from build123d import *

# Parameters (mm, degrees)
BASE_FLANGE1_DEPTH = 20
FILLET1_R          = 3
SKETCH2_R          = 1.5
CUT_EXTRUDE1_DEPTH = 3


# Sheet-metal steps are written as plain solids
with BuildPart() as part:
    # Sketch1 → Base-Flange1 (new body)
    with BuildSketch(Plane(origin=(0, 0, 0), x_dir=(0, 0, -1), z_dir=(1, 0, 0))):
        with BuildLine():
            Line((0, 0), (9.2634, 0))
            ThreePointArc((9.2634, 0), (9.784254855, 0.215745145), (10, 0.7366))
            Line((10, 0.7366), (10, 10))
            Line((10, 10), (13, 10))
            Line((13, 10), (13, 0.7366))
            ThreePointArc((13, 0.7366), (11.905575199, -1.905575199), (9.2634, -3))
            Line((9.2634, -3), (0, -3))
            Line((0, -3), (0, 0))
        make_face()
    extrude(amount=BASE_FLANGE1_DEPTH)

    # Fillet1
    fillet1_edges = [part.edges().sort_by_distance(p)[0] for p in [
        (20, -1.5, 0),
        (20, 10, -11.5),
        (0, -1.5, 0),
        (0, 10, -11.5),
    ]]
    fillet(fillet1_edges, radius=FILLET1_R)

    # Sketch2 → Cut-Extrude1 (cut)
    with BuildSketch(Plane(origin=(0, 0, -13), x_dir=(-1, 0, 0), z_dir=(0, 0, -1))):
        with Locations((-10, 2.5)):
            Circle(SKETCH2_R)
    extrude(amount=-CUT_EXTRUDE1_DEPTH, mode=Mode.SUBTRACT)


solid = part.part
Part model, mm, in its own coordinate system. A direction names the side the tool comes from. Coordinates: 2 decimals unless noted, no trailing zeros. Write each loop counter-clockwise with the first axis right and the second up, starting at its lowest first coordinate (ties: lowest second). Pieces come first, ordered by that corner, then holes. Notation, with made-up numbers: (-26, -30) - (4, -30) arc R18 ccw to (4, -26) - close; hole circle Ø9 at (-10, 2). An arc over 180 degrees is marked (long way). Put each result on its own line as item: value.
1. Band-saw the part on B-B (y = 2.5). Write the cut outline in (x, z), then the cut area to 3 significant figures.
Final values:
outline: (0, -13) - (8.5, -13) - (8.5, -10) - (0, -10) - close; (11.5, -13) - (20, -13) - (20, -10) - (11.5, -10) - close
area: 51.0 mm²
2. Band-saw the part on D-D (y = 4.5). Write the cut outline in (x, z), then the cut area to 3 significant figures.
Final values:
outline: (0, -13) - (20, -13) - (20, -10) - (0, -10) - close
area: 60.0 mm²
3. Flat gauge pins, fed straight in: pin 1 Ø7.5 at (x, z) = (9.5, -4.5) entering from +Y; pin 2 Ø3.5 at (x, y) = (10, 2.5) entering from +Z. Where does each tip first touch, or does it go through?
Final values:
pin 1: stops at y = 0
pin 2: stops at z = -10
4. Band-saw the part on A-A (x = 10). Write the cut outline in (y, z).
Final values:
outline: (-3, -9.26) arc R3.74 ccw to (0.74, -13) - (1, -13) - (1, -10) - (0.74, -10) arc R0.74 cw to (0, -9.26) - (0, 0) - (-3, 0) - close; (4, -13) - (10, -13) - (10, -10) - (4, -10) - close
5. 3-axis set-ups, long thin cutter, end or side, ignore diameter. For faces 1 (the flat face through (10, 5, -10)), 2 (the flat face through (10, -2, 0)): which of +Z, -Z, +X, -X, +Y, -Y reach the whole face in a straight line?
Final values:
face 1: +Z, +X, -X, +Y
face 2: +Z, +X, -X, +Y, -Y
6. Band-saw the part on C-C (x = 8). Write the cut outline in (y, z).
Final values:
outline: (-3, -9.26) arc R3.74 ccw to (0.74, -13) - (10, -13) - (10, -10) - (0.74, -10) arc R0.74 cw to (0, -9.26) - (0, 0) - (-3, 0) - close
7. Probe line 1 along Z through (x, y) = (14.5, 1.5); line 2 along Y through (x, z) = (10, -11); line 3 along Y through (x, z) = (10, -11.2). List the from-to ranges inside material, lowest first. Write a range as [from, to].
Final values:
line 1: z = [-13, -10]
line 2: y = [-2.57, 1], [4, 10]
line 3: y = [-2.46, 1], [4, 10]
8. Two-plate mould, pull along X, no slides. Class faces 3 (the flat face through (10, -3, -5)), 4 (the cylindrical face through (11.2, 1.6, -11.5)), 5 (the flat face through (0, 1, -10.3)), 6 (the cylindrical face through (19.1, -1.48, -0.86)): +X half, -X half, draft (parallel to the pull), parting line (faces both ways), or undercut.
Final values:
face 3: draft
face 4: undercut
face 5: -X half
face 6: +X half
